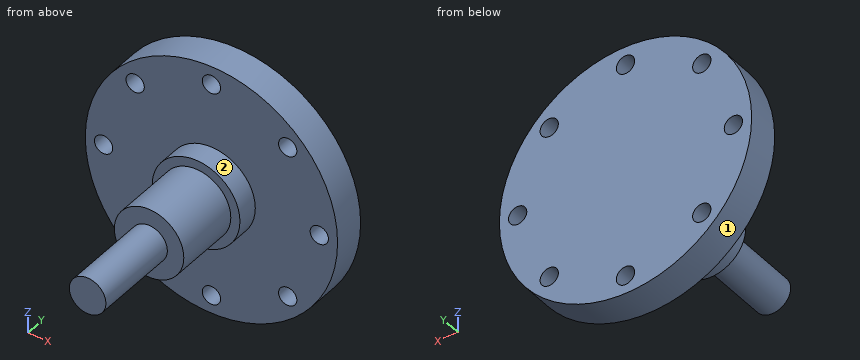
```python
from build123d import *

# Parameters (mm, degrees)
CROQUIS1_R              = 17.25
CROQUIS1_R_2            = 1.25
SALIENTE_EXTRUIR1_DEPTH = 4.5
CROQUIS3_R              = 4.75
SALIENTE_EXTRUIR3_DEPTH = 12.175
CROQUIS4_R              = 6
SALIENTE_EXTRUIR4_DEPTH = 3
CROQUIS5_R              = 2.5
SALIENTE_EXTRUIR5_DEPTH = 12


with BuildPart() as part:
    # Croquis1 → Saliente-Extruir1 (new body)
    with BuildSketch(Plane(origin=(0, 0, 0), x_dir=(1, 0, 0), z_dir=(0, 1, 0))):
        Circle(CROQUIS1_R)
        with Locations((14.75, 0)):
            Circle(CROQUIS1_R_2, mode=Mode.SUBTRACT)
        with Locations((10.429825023, -10.429825023)):
            Circle(CROQUIS1_R_2, mode=Mode.SUBTRACT)
        with Locations((0, -14.75)):
            Circle(CROQUIS1_R_2, mode=Mode.SUBTRACT)
        with Locations((-10.429825023, -10.429825023)):
            Circle(CROQUIS1_R_2, mode=Mode.SUBTRACT)
        with Locations((-14.75, 0)):
            Circle(CROQUIS1_R_2, mode=Mode.SUBTRACT)
        with Locations((-10.429825023, 10.429825023)):
            Circle(CROQUIS1_R_2, mode=Mode.SUBTRACT)
        with Locations((0, 14.75)):
            Circle(CROQUIS1_R_2, mode=Mode.SUBTRACT)
        with Locations((10.429825023, 10.429825023)):
            Circle(CROQUIS1_R_2, mode=Mode.SUBTRACT)
    extrude(amount=SALIENTE_EXTRUIR1_DEPTH)

    # Croquis3 → Saliente-Extruir3 (add)
    with BuildSketch(Plane.XZ):
        Circle(CROQUIS3_R)
    extrude(amount=SALIENTE_EXTRUIR3_DEPTH)

    # Croquis4 → Saliente-Extruir4 (add)
    with BuildSketch(Plane.XZ):
        Circle(CROQUIS4_R)
    extrude(amount=SALIENTE_EXTRUIR4_DEPTH)

    # Croquis5 → Saliente-Extruir5 (add)
    with BuildSketch(Plane.XZ.offset(12.175)):
        Circle(CROQUIS5_R)
    extrude(amount=SALIENTE_EXTRUIR5_DEPTH)


solid = part.part
```
Here's how the part is built. I have some questions about the finished solid (model axes, mm). Face numbers are marked on the shaded views. A direction names the side the tool comes from. Round coordinates to 2 decimals unless told otherwise and drop trailing zeros. Order: outer loops, then holes, each group sorted by start corner. A loop starts at its lowest first (then second) coordinate and runs counter-clockwise, first axis right, second up. Notation, with made-up numbers: (76.5, 61) -> (85.5, 61) arc R14 cw to (85.5, 73) -> close; hole circle Ø4 at (-12.5, 45.5). An arc over 180 degrees is marked (long way). Use a Markdown table: item, result. Add a question column.
(1) I need wall thicknesses on line 1 along Z through (x, y) = (0, 2.9); line 2 along Y through (x, z) = (7, -13.5). Which ranges of each line are inside material? Lowest first, please.
(2) For pin 1 Ø10 at (x, z) = (-8, -10) entering from -Y; pin 2 Ø6 at (x, y) = (-1.5, -2.5) entering from +Z; pin 3 Ø6 at (x, y) = (12, 0.5) entering from -Z; pin 4 Ø1 at (y, z) = (-5, -3.5) entering from -X, each with a flat end and sliding along its axis, tell me the tip position at first contact or that it passes through.
(3) Suppose I cut it at B-B, the plane z = 0. Please give me the cut outline in (x, y) (3 decimals), and give its area (3 significant figures).
(4) Suppose I cut it at C-C, the plane x = -14.75. Please give me the cut outline in (y, z).
(5) For the marked faces 1 and 2, which set-ups out of +Z, -Z, +X, -X, +Y, -Y let a thin tool reach every point of the face, with its end or its side?
(6) Suppose I cut it at A-A, the plane x = 0. Please give me the cut outline in (y, z) (3 decimals).
(7) Suppose I cut it at D-D, the plane z = -14.75. Please give me the cut outline in (x, y), and give its area (3 significant figures).
Verdict:
| question | item | result |
|---|---|---|
| 1 | line 1 | -17.25 to -16, -13.5 to 13.5, 16 to 17.25 |
| 1 | line 2 | 0 to 4.5 |
| 2 | pin 1 | y = 0 |
| 2 | pin 2 | z = 17.25 |
| 2 | pin 3 | z = -14.72 |
| 2 | pin 4 | x = -3.68 |
| 3 | outline | (-17.25, 0) -> (-16, 0) -> (-16, 4.5) -> (-17.25, 4.5) -> close; (-13.5, 0) -> (-6, 0) -> (-6, -3) -> (-4.75, -3) -> (-4.75, -12.175) -> (-2.5, -12.175) -> (-2.5, -24.175) -> (2.5, -24.175) -> (2.5, -12.175) -> (4.75, -12.175) -> (4.75, -3) -> (6, -3) -> (6, 0) -> (13.5, 0) -> (13.5, 4.5) -> (-13.5, 4.5) -> close; (16, 0) -> (17.25, 0) -> (17.25, 4.5) -> (16, 4.5) -> close |
| 3 | area | 316 mm2 |
| 4 | outline | (0, -8.94) -> (4.5, -8.94) -> (4.5, -1.25) -> (0, -1.25) -> close; (0, 1.25) -> (4.5, 1.25) -> (4.5, 8.94) -> (0, 8.94) -> close |
| 5 | face 1 | +Y, -Y |
| 5 | face 2 | -Y |
| 6 | outline | (-24.175, -2.5) -> (-12.175, -2.5) -> (-12.175, -4.75) -> (-3, -4.75) -> (-3, -6) -> (0, -6) -> (0, -13.5) -> (4.5, -13.5) -> (4.5, 13.5) -> (0, 13.5) -> (0, 6) -> (-3, 6) -> (-3, 4.75) -> (-12.175, 4.75) -> (-12.175, 2.5) -> (-24.175, 2.5) -> close; (0, -17.25) -> (4.5, -17.25) -> (4.5, -16) -> (0, -16) -> close; (0, 16) -> (4.5, 16) -> (4.5, 17.25) -> (0, 17.25) -> close |
| 7 | outline | (-8.94, 0) -> (-1.25, 0) -> (-1.25, 4.5) -> (-8.94, 4.5) -> close; (1.25, 0) -> (8.94, 0) -> (8.94, 4.5) -> (1.25, 4.5) -> close |
| 7 | area | 69.2 mm2 |
